Source: CAD feature listing. Evaluate the final solid. Frame: model axes, mm. A direction names the side the tool comes from. Round coordinates to 2 decimals unless told otherwise and drop trailing zeros. Order: outer loops, then holes, each group sorted by start corner. A loop starts at its lowest first (then second) coordinate and runs counter-clockwise, first axis right, second up. Notation, with made-up numbers: (37, -27.75) -> (69, -27.75) arc R25 cw to (69, 7.25) -> close; hole circle Ø5 at (23.5, 17). An arc over 180 degrees is marked (long way). Write item = value, one per line. Start each with the question number.
(1) Cut plane C-C on z = 12.75. Return the cut outline in (x, y).
(2) Cut plane D-D on z = 5.25. Return the cut outline in (x, y).
(3) Cut plane A-A on x = 0. Return the cut outline in (y, z).
(4) Ray query, line 1 (Y direction, x = 2.5, z = 5); line 2 (Z direction, x = 2.25, y = -7.5); line 3 (X direction, y = 5.5, z = 4). Return the intervals inside material, ascending.
(5) Contact query for flat-ended pins moving along their axis: pin 1 Ø6 at (x, y) = (-0.5, -4.5) entering from -Z; pin 2 Ø5 at (y, z) = (-1.5, 12) entering from +X; pin 3 Ø1 at (x, z) = (4, 8.5) entering from -Y; pin 4 Ø1.5 at (y, z) = (-4, 13.5) entering from -X. Output: stop coordinate, or through.
(6) Draft query along X for faces 1 (the face through (-2.17, -9.76, 16.48)), 2 (the face through (0, 0, 12)), 3 (the face through (0, 0, 18)). Return one class per face: released by +X, released by -X, zero draft, split by the parting line, or undercut.
(7) Reachability of faces 4 (the face through (-3, 3, 0)), 5 (the face through (7, -2, 15)) from +Z, -Z, +X, -X, +Y, -Y: full face, straight path, thin tool, end or side. Return the list, or none.
from build123d import *

# Parameters (mm, degrees)
F2_R     = 10
F3_DEPTH = 3


with BuildPart() as f1:
    # F0 (on Front) → F1 (revolve)
    with BuildSketch(Plane.XZ):
        Polygon((2.05, 12), (3.55, 0), (6.55, 0), (6.55, 15), (0, 15), (0, 12), align=None)
    revolve(axis=Axis((0, 0, 3.882699), (0, 0, -1)))

    # F2 (on face) → F3 (join)
    with BuildSketch(Plane.XY.offset(15)):
        Circle(F2_R)
    extrude(amount=F3_DEPTH)


solid = f1.part
Evaluation:
q1.outline = circle Ø13.1 at (0, 0)
q2.outline = circle Ø13.1 at (0, 0); hole circle Ø5.79 at (0, 0)
q3.outline = (-10, 15) -> (-6.55, 15) -> (-6.55, 0) -> (-3.55, 0) -> (-2.05, 12) -> (2.05, 12) -> (3.55, 0) -> (6.55, 0) -> (6.55, 15) -> (10, 15) -> (10, 18) -> (-10, 18) -> close
q4.line_1 = -6.05 to -1.52, 1.52 to 6.05
q4.line_2 = 15 to 18
q4.line_3 = -3.56 to 3.56
q5.pin_1 = 0
q5.pin_2 = 6.55
q5.pin_3 = -5.54
q5.pin_4 = -5.69
q6.face_1 = split by the parting line
q6.face_2 = undercut
q6.face_3 = zero draft
q7.face_4 = -Z, +X, -X, +Y, -Y
q7.face_5 = -Z
